Could you check a few things on this drawing? It's one solid part, dimensions in mm from its lowest x, y, z. A direction names the side the tool comes from. Round coordinates to 2 decimals unless told otherwise and drop trailing zeros. Order: outer loops, then holes, each group sorted by start corner. A loop starts at its lowest first (then second) coordinate and runs counter-clockwise, first axis right, second up. Notation, with made-up numbers: (14, 73.25) -> (60, 73.25) arc R16 ccw to (60, 100.25) -> close; hole circle Ø6 at (24, 64). An arc over 180 degrees is marked (long way). Use a Markdown table: item, result. Add a question column.
(1) I want a section at C-C, the plane z = 11. Please give me the cut outline in (x, y).
(2) Thinking about a two-plate mould opening in Z: for the marked faces 1, 2, 3 and 4, which applies, pulls with the +Z half, pulls with the -Z half, needs draft (parallel to the pull), parting line crosses it, or undercut?
(3) I want a section at A-A, the plane x = 14.5. Please give me the cut outline in (y, z) (1 decimal).
(4) I want a section at D-D, the plane x = 18.5. Please give me the cut outline in (y, z) (1 decimal), then the cut area to 3 significant figures.
(5) On a 3-axis mill with a long thin cutter (end or side, diameter ignored), from which of +Z, -Z, +X, -X, +Y, -Y can I reach the whole of each face in a straight line? I mean the marked faces 5, 6 and 7. Say none if no direction works.
(6) I'm going to push flat-ended pins straight in: P1, Ø2.5, axis at y = 24, z = 2.5, coming from the -X side; P2, Ø4, axis at y = 4, z = 12, coming from the -X side; P3, Ø5, axis at x = 8, z = 8.5, coming from the -Y side; P4, Ø1.5, axis at y = 27, z = 9.5, coming from the +X side. Where does each tip first touch, or does it pass through?
(7) I want a section at B-B, the plane y = 25.75. Please give me the cut outline in (x, z), then the cut area to 3 significant figures.
(8) If I drill on probe 1 along Z at (x, y) = (24.5, 24); probe 2 along Y at (x, z) = (9, 20); probe 3 along Y at (x, z) = (14.5, 3.75) (1 decimal), over which ranges is the centre line in solid material (lowest first)?
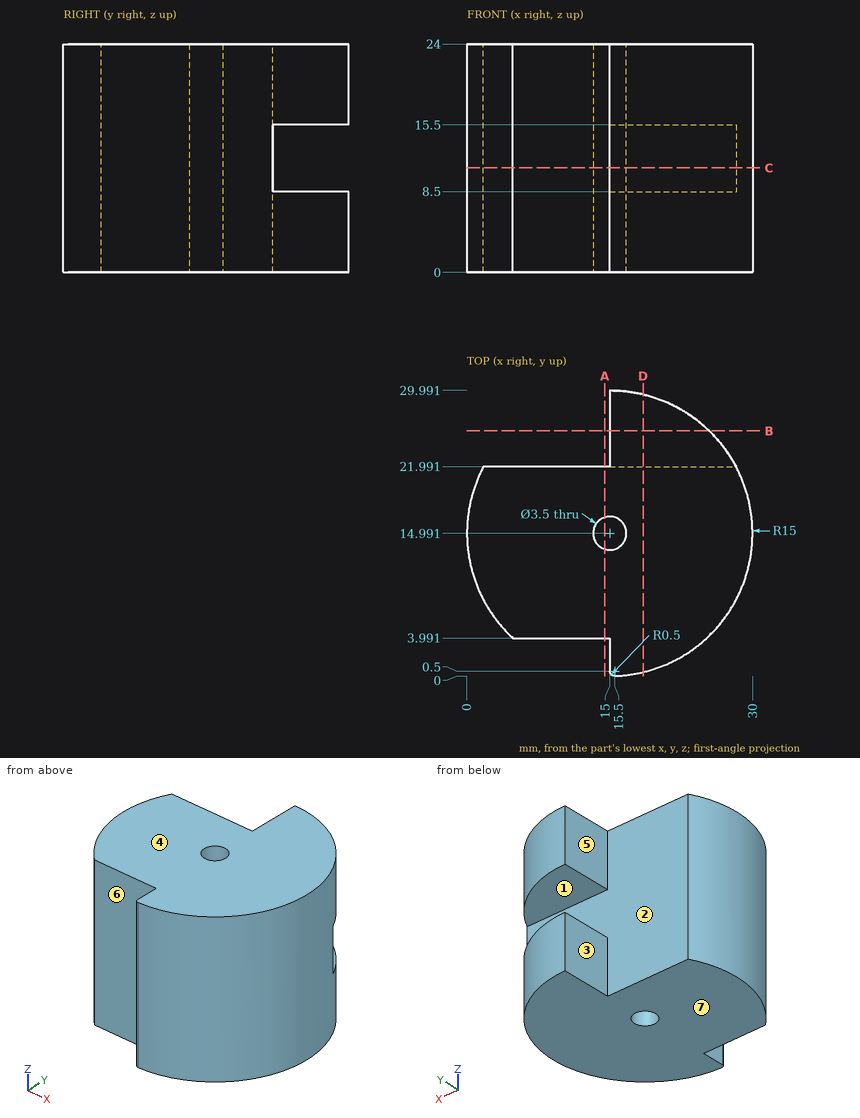
Taken from the geometry:
| question | item | result |
|---|---|---|
| 1 | outline | (1.73, 21.99) arc R15 ccw to (4.8, 3.99) -> (15, 3.99) -> (15, 0.5) arc R0.5 ccw to (15.52, 0) arc R15 ccw to (28.27, 21.99) -> close; hole circle Ø3.5 at (15, 14.99) |
| 2 | face 1 | undercut |
| 2 | face 2 | undercut |
| 2 | face 3 | needs draft |
| 2 | face 4 | pulls with the +Z half |
| 3 | outline | (4, 0) -> (13.3, 0) -> (13.3, 24) -> (4, 24) -> close; (16.7, 0) -> (22, 0) -> (22, 24) -> (16.7, 24) -> close |
| 4 | outline | (0.4, 0) -> (29.6, 0) -> (29.6, 8.5) -> (22, 8.5) -> (22, 15.5) -> (29.6, 15.5) -> (29.6, 24) -> (0.4, 24) -> close |
| 4 | area | 647 mm2 |
| 5 | face 5 | +Z, -Z, -X, +Y |
| 5 | face 6 | +Z, -Z, -X, -Y |
| 5 | face 7 | -Z, +X, -X, +Y, -Y |
| 6 | P1 | stops at x = 15 |
| 6 | P2 | stops at x = 2.99 |
| 6 | P3 | stops at y = 3.99 |
| 6 | P4 | passes through |
| 7 | outline | (15, 0) -> (25.45, 0) -> (25.45, 8.5) -> (15, 8.5) -> close; (15, 15.5) -> (25.45, 15.5) -> (25.45, 24) -> (15, 24) -> close |
| 7 | area | 178 mm2 |
| 8 | probe 1 | z = 0 to 8.5, 15.5 to 24 |
| 8 | probe 2 | y = 3.99 to 21.99 |
| 8 | probe 3 | y = 4 to 13.3, 16.7 to 22 |
